from build123d import *

# Parameters (mm, degrees)
F1_DEPTH = 15
F2_DEPTH = 13
F3_DEPTH = 1.2
F4_DEPTH = 25
F5_DEPTH = 4


with BuildPart() as f1:
    # F0 (on Top) → F1 (new body)
    with BuildSketch(Plane.XY):
        with BuildLine():
            ThreePointArc((-3, 17.2409396496), (0, 17.5), (3, 17.2409396496))
            Line((3, 17.2409396496), (3, 18.6603858481))
            ThreePointArc((3, 18.6603858481), (0, 18.9), (-3, 18.6603858481))
            Line((-3, 18.6603858481), (-3, 17.2409396496))
        make_face()
        with BuildLine():
            Line((3, 18.6603858481), (3, 17.2409396496))
            ThreePointArc((3, 17.2409396496), (13.393095236, 11.2638803261), (17.5, 0))
            ThreePointArc((17.5, 0), (-11.2638803261, -13.393095236), (-3, 17.2409396496))
            Line((-3, 17.2409396496), (-3, 18.6603858481))
            ThreePointArc((-3, 18.6603858481), (-12.2578546247, -14.3859306268), (18.9, 0))
            ThreePointArc((18.9, 0), (14.3859306268, 12.2578546247), (3, 18.6603858481))
        make_face()
        with BuildLine():
            ThreePointArc((-3, 13.6747943312), (0, 14), (3, 13.6747943312))
            Line((3, 13.6747943312), (3, 17.2409396496))
            ThreePointArc((3, 17.2409396496), (0, 17.5), (-3, 17.2409396496))
            Line((-3, 17.2409396496), (-3, 13.6747943312))
        make_face()
        with BuildLine():
            ThreePointArc((3, 13.6747943312), (10.9087121146, 8.7749643874), (14, 0))
            ThreePointArc((14, 0), (-8.7749643874, -10.9087121146), (-3, 13.6747943312))
            Line((-3, 13.6747943312), (-3, 17.2409396496))
            ThreePointArc((-3, 17.2409396496), (-11.2638803261, -13.393095236), (17.5, 0))
            ThreePointArc((17.5, 0), (13.393095236, 11.2638803261), (3, 17.2409396496))
            Line((3, 17.2409396496), (3, 13.6747943312))
        make_face()
    extrude(amount=F1_DEPTH)

    # F0 (on Top) → F2 (cut)
    with BuildSketch(Plane.XY):
        with BuildLine():
            ThreePointArc((-3, 13.6747943312), (0, 14), (3, 13.6747943312))
            Line((3, 13.6747943312), (3, 17.2409396496))
            ThreePointArc((3, 17.2409396496), (0, 17.5), (-3, 17.2409396496))
            Line((-3, 17.2409396496), (-3, 13.6747943312))
        make_face()
        with BuildLine():
            ThreePointArc((3, 13.6747943312), (10.9087121146, 8.7749643874), (14, 0))
            ThreePointArc((14, 0), (-8.7749643874, -10.9087121146), (-3, 13.6747943312))
            Line((-3, 13.6747943312), (-3, 17.2409396496))
            ThreePointArc((-3, 17.2409396496), (-11.2638803261, -13.393095236), (17.5, 0))
            ThreePointArc((17.5, 0), (13.393095236, 11.2638803261), (3, 17.2409396496))
            Line((3, 17.2409396496), (3, 13.6747943312))
        make_face()
    extrude(amount=F2_DEPTH, mode=Mode.SUBTRACT)

    # F0 (on Top) → F3 (join)
    with BuildSketch(Plane.XY):
        with BuildLine():
            ThreePointArc((-3, 18.6603858481), (0, 18.9), (3, 18.6603858481))
            Line((3, 18.6603858481), (3, 47.4051684946))
            ThreePointArc((3, 47.4051684946), (0, 47.5), (-3, 47.4051684946))
            Line((-3, 47.4051684946), (-3, 18.6603858481))
        make_face()
        with BuildLine():
            Line((3, 47.4051684946), (3, 18.6603858481))
            ThreePointArc((3, 18.6603858481), (14.3859306268, 12.2578546247), (18.9, 0))
            ThreePointArc((18.9, 0), (-12.2578546247, -14.3859306268), (-3, 18.6603858481))
            Line((-3, 18.6603858481), (-3, 47.4051684946))
            ThreePointArc((-3, 47.4051684946), (-32.5096139626, -34.6319938785), (47.5, 0))
            ThreePointArc((47.5, 0), (34.6319938785, 32.5096139626), (3, 47.4051684946))
        make_face()
    extrude(amount=F3_DEPTH)

    # F0 (on Top) → F4 (join)
    with BuildSketch(Plane.XY):
        with BuildLine():
            ThreePointArc((-3, 47.4051684946), (0, 47.5), (3, 47.4051684946))
            Line((3, 47.4051684946), (3, 49.9099188539))
            ThreePointArc((3, 49.9099188539), (0, 50), (-3, 49.9099188539))
            Line((-3, 49.9099188539), (-3, 47.4051684946))
        make_face()
        with BuildLine():
            Line((3, 49.9099188539), (3, 47.4051684946))
            ThreePointArc((3, 47.4051684946), (34.6319938785, 32.5096139626), (47.5, 0))
            ThreePointArc((47.5, 0), (-32.5096139626, -34.6319938785), (-3, 47.4051684946))
            Line((-3, 47.4051684946), (-3, 49.9099188539))
            ThreePointArc((-3, 49.9099188539), (-34.278273002, -36.4005494464), (50, 0))
            ThreePointArc((50, 0), (36.4005494464, 34.278273002), (3, 49.9099188539))
        make_face()
    extrude(amount=F4_DEPTH)

    # F0 (on Top) → F5 (cut)
    with BuildSketch(Plane.XY):
        with BuildLine():
            ThreePointArc((-3, 17.2409396496), (0, 17.5), (3, 17.2409396496))
            Line((3, 17.2409396496), (3, 18.6603858481))
            ThreePointArc((3, 18.6603858481), (0, 18.9), (-3, 18.6603858481))
            Line((-3, 18.6603858481), (-3, 17.2409396496))
        make_face()
        with BuildLine():
            ThreePointArc((-3, 18.6603858481), (0, 18.9), (3, 18.6603858481))
            Line((3, 18.6603858481), (3, 47.4051684946))
            ThreePointArc((3, 47.4051684946), (0, 47.5), (-3, 47.4051684946))
            Line((-3, 47.4051684946), (-3, 18.6603858481))
        make_face()
        with BuildLine():
            ThreePointArc((-3, 47.4051684946), (0, 47.5), (3, 47.4051684946))
            Line((3, 47.4051684946), (3, 49.9099188539))
            ThreePointArc((3, 49.9099188539), (0, 50), (-3, 49.9099188539))
            Line((-3, 49.9099188539), (-3, 47.4051684946))
        make_face()
    extrude(amount=F5_DEPTH, mode=Mode.SUBTRACT)


solid = f1.part
Source: CAD feature listing. Evaluate the final solid. Frame: model axes, mm. A direction names the side the tool comes from. Round coordinates to 2 decimals unless told otherwise and drop trailing zeros. Loops run counter-clockwise (first coordinate to the right, second up) from the corner with the lowest first, then second, coordinate; pieces in that order, holes last.
Q1. Mould query, pull axis X, two halves, no side actions, for faces 4 (the face through (-8, 12, 13)), 5 (the face through (3, 37, 1)), 6 (the face through (18.3, -44.2, 25)). Classes: pulls with the +X half, pulls with the -X half, needs draft (parallel to the pull), parting line crosses it, or undercut.
Q2. Section B-B, the plane z = 9.25. Return loops of the section in (x, y), plus the area to 3 significant figures.
Q3. Section A-A, the plane x = 0. Return loops of the section in (y, z).
Q4. Access query for faces 1 (the face through (-13, -7, 15)), 2 (the face through (-3, 37, 1)), 3 (the face through (-1, -22, 0)). Directions: +Z, -Z, +X, -X, +Y, -Y. A direction counts if a zero-diameter tool reaches every point of the face in a straight line with its end or side. Return the directions, or none.
Q5. Ray query, line 1 (Y direction, x = 0, z = 13.5); line 2 (X direction, y = 1, z = 7.5). Return the intervals inside material, ascending.
Q6. Section C-C, the plane z = 21.75. Return loops of the section in (x, y).
Q7. First-contact query: P1, Ø12, axis at y = 12.5, z = 8.5, coming from the +X side; P2, Ø12, axis at x = -8.5, z = 21.5, coming from the -Y side; P3, Ø1, axis at y = -5, z = 15.5, coming from the +X side. Flat tips, straight axial feed; report the tip coordinate or a pass-through.
Q8. Section D-D, the plane x = -20.5. Return loops of the section in (y, z), plus the area to 3 significant figures.
Solutions:
1. face 4: undercut
1. face 5: undercut
1. face 6: needs draft
2. outline: circle Ø100 at (0, 0); circle Ø37.8 at (0, 0); hole circle Ø95 at (0, 0); hole circle Ø35 at (0, 0)
2. area: 926 mm2
3. outline: (-50, 0) - (-17.5, 0) - (-17.5, 13) - (-14, 13) - (-14, 15) - (-18.9, 15) - (-18.9, 1.2) - (-47.5, 1.2) - (-47.5, 25) - (-50, 25) - close; (14, 13) - (17.5, 13) - (17.5, 4) - (18.9, 4) - (18.9, 15) - (14, 15) - close; (47.5, 4) - (50, 4) - (50, 25) - (47.5, 25) - close
4. face 1: +Z
4. face 2: -Z, +Y
4. face 3: -Z, +X, -X, +Y, -Y
5. line 1: y = -50 to -47.5, -18.9 to -14, 14 to 18.9, 47.5 to 50
5. line 2: x = -49.99 to -47.49, -18.87 to -17.47, 17.47 to 18.87, 47.49 to 49.99
6. outline: circle Ø100 at (0, 0); hole circle Ø95 at (0, 0)
7. P1: stops at x = 49.58
7. P2: stops at y = -49.94
7. P3: stops at x = 49.8
8. outline: (-45.6, 0) - (45.6, 0) - (45.6, 25) - (42.85, 25) - (42.85, 1.2) - (-42.85, 1.2) - (-42.85, 25) - (-45.6, 25) - close
8. area: 241 mm2
